The figure shows three views and two pictorial views of one solid part (mm, origin at its lowest corner). Answer the questions. Round coordinates to 2 decimals unless told otherwise and drop trailing zeros. Order: outer loops, then holes, each group sorted by start corner. A loop starts at its lowest first (then second) coordinate and runs counter-clockwise, first axis right, second up. Notation, with made-up numbers: (42.25, -27.75) -> (101.25, -27.75) arc R5 ccw to (101.25, -23.75) -> close; hole circle Ø10 at (43.25, 58). An arc over 180 degrees is marked (long way). Return JSON: item names as keys, results as strings. Group by question number.
(1) The part is cut by section A-A (x = 87). Determine the outline of the cut face in (y, z), plus the area to 3 significant figures.
(2) The part is cut by section B-B (y = 1628). Determine the outline of the cut face in (x, z).
(3) Each of these flat-tipped pins is pushed along its axis until it touches: pin 1 (1.5 mm diameter, centred on x = 117, z = 33, fed in from +Y); pin 2 (5 mm diameter, centred on x = 20, y = 1579.5, fed in from +Z); pin 3 (12 mm diameter, centred on x = 76, y = 672, fed in from -Z); pin 4 (2 mm diameter, centred on x = 78, z = 23, fed in from -Y). Where does it stop, or does it pass through?
(4) Consider line 1 (X direction, y = 1900.5, z = 42); line 2 (X direction, y = 1176, z = 6.5); line 3 (Y direction, x = 100.5, z = 24). Determine where each line is inside the solid, lowest interval first. Write a range as [from, to].
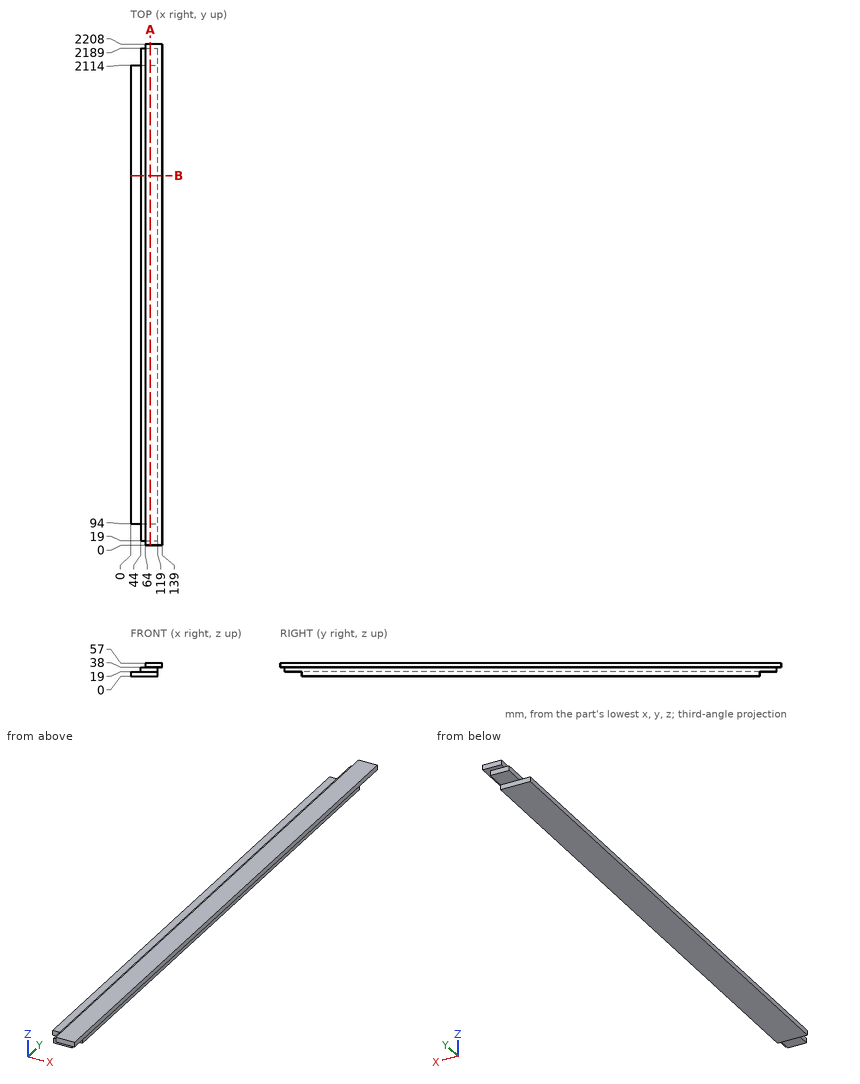
Answer below:
{
 "1": {"outline": "(0, 38) -> (19, 38) -> (19, 19) -> (94, 19) -> (94, 0) -> (2114, 0) -> (2114, 19) -> (2189, 19) -> (2189, 38) -> (2208, 38) -> (2208, 57) -> (0, 57) -> close", "area": "122,000 mm²"},
 "2": {"outline": "(0, 0) -> (119, 0) -> (119, 38) -> (139, 38) -> (139, 57) -> (64, 57) -> (64, 38) -> (44, 38) -> (44, 19) -> (0, 19) -> close"},
 "3": {"pin 1": "stops at y = 2189", "pin 2": "stops at z = 19", "pin 3": "stops at z = 0", "pin 4": "stops at y = 19"},
 "4": {"line 1": "x = [64, 139]", "line 2": "x = [0, 119]", "line 3": "y = [19, 2189]"}
}
